Input: part model. Units: mm. Frame: model coordinates. Coordinates: 2 decimals unless noted, no trailing zeros. Loops run counter-clockwise (first coordinate to the right, second up) from the corner with the lowest first, then second, coordinate; pieces in that order, holes last. Notation, with made-up numbers: (43, -34) -> (77, -34) arc R8 cw to (77, -30) -> close; hole circle Ø6 at (2, 70). An arc over 180 degrees is marked (long way). Answer as a JSON object with one key per item and string values.
Autodesk Inventor part; units mm, degrees
ref_plane "YZ Plane" through (0, 0, 0) normal (1, 0, 0) x (0, 1, 0)
ref_plane "XZ Plane" through (0, 0, 0) normal (0, 1, 0) x (-1, 0, 0)
ref_plane "XY Plane" through (0, 0, 0) normal (0, 0, 1) x (1, 0, 0)
ref_plane "Work Plane1" through (678.6266, 4, 0) normal (0, 0, 1) x (1, 0, 0)
sketch "Sketch1" plane through (678.6266, 4, 0) normal (0, 0, 1) x (1, 0, 0)
  circle A0 centre (-710.3818, -172.4297) radius 4.25
  line L0 (-690.3818, -322.4297) -> (-513.3818, -322.4297) construction
  circle A1 centre (-679.3818, -145.4297) radius 5
  circle A2 centre (-619.3818, -145.4297) radius 5
  line L1 (-730.3818, -322.4297) -> (-695.3818, -322.4297)
  line L2 (-695.3818, -322.4297) -> (-695.3818, -232.4297)
  line L3 (-695.3818, -232.4297) -> (-603.3818, -232.4297)
  line L4 (-603.3818, -232.4297) -> (-603.3818, -322.4297)
  circle A3 centre (-710.3818, -172.4297) radius 4.25
  circle A4 centre (-513.3818, -292.4297) radius 4.25
  circle A5 centre (-510.3818, -60.4297) radius 4.25
  line L5 (-488.3818, -194.7007) -> (-492.3818, -194.7007)
  line L6 (-492.3818, -194.7007) -> (-492.3818, -322.4297)
  line L7 (-492.3818, -322.4297) -> (-492.3818, -22.4297)
  line L8 (-492.3818, -322.4297) -> (-603.3818, -322.4297)
  line L9 (-555.3818, -22.4297) -> (-492.3818, -22.4297)
  line L10 (-492.3818, -22.4297) -> (-560.3818, -22.4297)
  line L11 (-560.3818, -22.4297) -> (-560.3818, -120.4297)
  circle A6 centre (-710.3818, -297.4297) radius 4.25
  line L12 (-560.3818, -22.4297) -> (-560.3818, -122.4297)
  line L13 (-560.3818, -122.4297) -> (-730.3818, -122.4297)
  line L14 (-730.3818, -322.4297) -> (-730.3818, -122.4297)
  line L15 (-710.3818, -122.4297) -> (-710.3818, -182.4297)
  line L16 (-710.3818, -182.4297) -> (-596.3818, -182.4297)
  line L17 (-596.3818, -182.4297) -> (-596.3818, -122.4297)
  circle A7 centre (-710.3818, -172.4297) radius 7
  circle A8 centre (-709.3818, -258.4297) radius 5.25
  circle A9 centre (-709.3818, -212.4297) radius 5.25
  line L18 (-709.3818, -258.4297) -> (-589.3818, -258.4297) construction
  circle A10 centre (-589.3818, -258.4297) radius 5.25
  circle A11 centre (-589.3818, -212.4297) radius 5.25
  point P0 (-678.6266, -4)
  dimension "d52" = 8.5
  dimension "d57" = 10
  dimension "d59" = 10
  dimension "d61" = 35
  dimension "d62" = 92
  dimension "d70" = 8.5
  dimension "d71" = 8.5
  dimension "d72" = 4
  dimension "d73" = 68
  dimension "d75" = 8.5
  dimension "d76" = 100
  dimension "d77" = 200
  dimension "d78" = 170
  dimension "d80" = 60
  dimension "d81" = 114
  dimension "d88" = 14
  dimension "d95" = 10.5
  dimension "d96" = 10.5
  dimension "d100" = 10.5
  dimension "d101" = 10.5
extrude "Extrusion5" add sketch "Sketch1" against normal blind 10 contours A0 L15 | A0 L15 A7 | L15 A0 | A0 L15 A7 | A7 L15 L16 L17 L13 L12 L11 L10 L9 L7 L6 L8 L4 L3 L2 L1 L14 | L15 L13 L17 L16 A7 | A8 | A9 | A10 | A11
extrude "Extrusion7" cut sketch "Sketch1" against normal blind 1.5 contours A0 L15 | A0 L15 A7 | L15 L13 L17 L16 A7 picked at (-708.9651, -172.4297) picked at (-709.5473, -178.419)
extrude "Extrusion6" cut sketch "Sketch1" against normal blind 10 contours A0 L15 | L15 A0
extrude "Extrusion8" cut sketch "Sketch1" against normal blind 1.5 contours A0 L15 A7 | A0 L15 A7
extrude "Extrusion9" cut sketch "Sketch1" against normal blind 10.5 contours A8 | A9 | A10 | A11
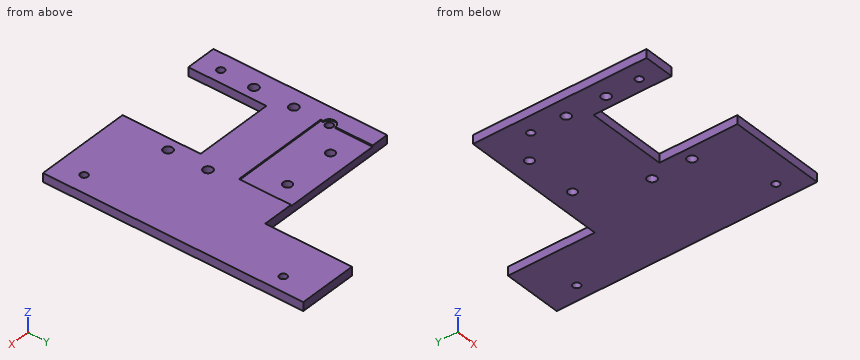
1. Section query D-D (y = -89.5). Return loops of the section in (x, z).
Reply:
{"outline": "(118.24, -10) -> (186.24, -10) -> (186.24, 0) -> (118.24, 0) -> close"}
2. Section query B-B (z = -6.5). Count the separate pieces of the cut face and the enclosed holes in it, plus the area to 3 significant figures.
Reply:
{"separate pieces": "1", "enclosed holes": "10", "area": "45,400 mm2"}
3. Pin query (flat end, axial travel): P1, Ø11.5, axis at x = -0.76, y = -141.43, coming from the +Z side; P2, Ø8.5, axis at x = -30.76, y = -208.43, coming from the +Z side; P3, Ø4, axis at y = -89.5, z = -5, coming from the -X side; P4, Ø5, axis at x = 51.5, z = -6, coming from the +Y side. Return the tip coordinate at first contact, or that it passes through.
Reply:
{"P1": "stops at z = -1.5", "P2": "passes through", "P3": "stops at x = 118.24", "P4": "stops at y = -118.43"}
4. Section query C-C (x = 18.5). Return loops of the section in (y, z), plus the area to 3 significant figures.
Reply:
{"outline": "(-228.43, -10) -> (-118.43, -10) -> (-118.43, -1.5) -> (-178.43, -1.5) -> (-178.43, 0) -> (-228.43, 0) -> close", "area": "1,010 mm2"}
5. Section query A-A (y = -238). Return loops of the section in (x, z).
Reply:
{"outline": "(-51.76, -10) -> (-16.76, -10) -> (-16.76, 0) -> (-51.76, 0) -> close; (75.24, -10) -> (186.24, -10) -> (186.24, 0) -> (75.24, 0) -> close"}
6. Line query: line 1 along Y through (x, z) = (91, -6.25); line 2 along X through (y, z) = (-138, -9); line 3 along X through (y, z) = (-139.5, -7.5). Output: solid intervals per line, ascending.
Reply:
{"line 1": "y = -318.43 to -259.38, -249.48 to -213.38, -203.48 to -118.43", "line 2": "x = -51.76 to -4.39, 2.88 to 55.61, 62.88 to 186.24", "line 3": "x = -51.76 to -5.37, 3.86 to 54.63, 63.86 to 186.24"}
